Check sheet for the modelled part. Datum: model origin and axes. Units: mm. Face numbers are marked on the shaded views. A direction names the side the tool comes from. Coordinates: 2 decimals unless noted, no trailing zeros. Loops run counter-clockwise (first coordinate to the right, second up) from the corner with the lowest first, then second, coordinate; pieces in that order, holes last. Notation, with made-up numbers: M 76,-37.75 L 87,-37.75 A36 cw 87,1.25 Z; hole C 54.25,66 d4. An arc over 180 degrees is marked long. Return JSON: item names as keys, results as strings.
from build123d import *

# Parameters (mm, degrees)
SKETCH_W        = 50
SKETCH_H        = 50
SKETCH_R        = 4.56572
PAD_DEPTH       = 20
SKETCH001_W     = 35.718838
SKETCH001_H     = 17.102667
POCKET_DEPTH    = 10
POCKET001_DEPTH = 10


with BuildPart() as part:
    # Sketch → Pad (new body)
    with BuildSketch(Plane.XY):
        Rectangle(SKETCH_W, SKETCH_H)
        with Locations((-12.739399, -12.190962)):
            Circle(SKETCH_R, mode=Mode.SUBTRACT)
    extrude(amount=-PAD_DEPTH)

    # Sketch001 → Pocket (cut)
    with BuildSketch(Plane.XY):
        with Locations((-0.828983, 8.449547)):
            Rectangle(SKETCH001_W, SKETCH001_H)
    extrude(amount=-POCKET_DEPTH, mode=Mode.SUBTRACT)

    # Sketch002 → Pocket001 (cut)
    with BuildSketch(Plane.XY):
        with BuildLine():
            ThreePointArc((10.613772, -5.440841), (3.942315, -5.985276), (4.48675, -12.656733))
            Line((4.48675, -12.656733), (12.984974, -19.872584))
            ThreePointArc((12.984974, -19.872584), (19.656431, -19.328148), (19.111996, -12.656692))
            Line((10.613772, -5.440841), (19.111996, -12.656692))
        make_face()
    extrude(amount=-POCKET001_DEPTH, mode=Mode.SUBTRACT)


with BuildPart() as part_1:
    # Clone placement: moved
    add(part.part.moved(Location((25, 25, 0))))


solid = part_1.part
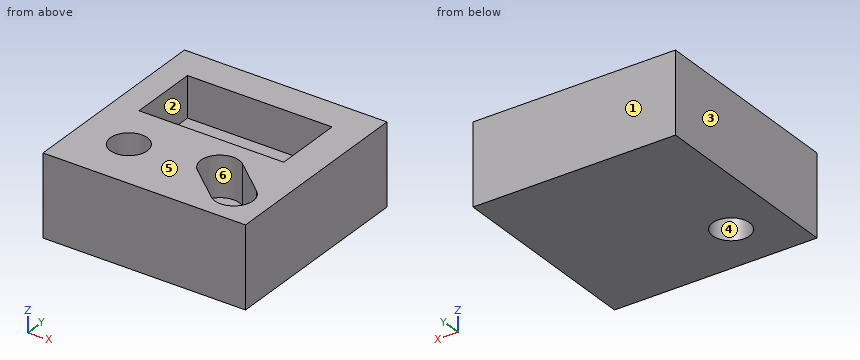
1) Section check A-A on y = 9. Record the cut outline in (x, z).
Answers:
{"outline": "M 0,-20 L 9.74,-20 L 9.74,0 L 0,0 Z; M 14.78,-20 L 50,-20 L 50,0 L 45.77,0 L 45.77,-10 L 33.42,-10 L 33.42,0 L 14.78,0 Z"}
2) Section check B-B on z = -6.75. Record the cut outline in (x, y).
Answers:
{"outline": "M 0,0 L 50,0 L 50,50 L 0,50 Z; hole M 6.31,24.9 L 42.03,24.9 L 42.03,42 L 6.31,42 Z; hole C 12.26,12.81 d9.13; hole M 29.49,12.34 L 37.98,5.13 A4.73 ccw 44.11,12.34 L 35.61,19.56 A4.73 ccw Z"}
3) Set-up check for the marked faces 5 and 6: record each of +Z, -Z, +X, -X, +Y, -Y from which the full face is reachable in a straight line by a thin tool's end or side.
Answers:
{"face 5": "+Z, +X, -X, +Y, -Y", "face 6": "+Z"}
4) Scan lines: line 1 along Y through (x, z) = (12, -9.25); line 2 along Y through (x, z) = (6.5, -3.75); line 3 along Y through (x, z) = (30.5, -9). Record each from-to range of solid material in increasing order. Write a range as [from, to].
Answers:
{"line 1": "[0, 8.25], [17.37, 24.9], [42, 50]", "line 2": "[0, 24.9], [42, 50]", "line 3": "[0, 11.48], [20.22, 24.9], [42, 50]"}
5) Go/stop test with a flat-tipped pin: pin 1 Ø5 at (x, y) = (27.5, 31) entering from +Z. Record where the tip stops, or that it passes through.
Answers:
{"pin 1": "z = -10"}
6) Draft check along Y on the marked faces 1, 2, 3 and 4. Enter one of: +Y half, -Y half, draft (parallel to the pull), parting line (faces both ways), or undercut.
Answers:
{"face 1": "+Y half", "face 2": "undercut", "face 3": "draft", "face 4": "undercut"}
7) Section check D-D on x = 19. Record the cut outline in (y, z), then the cut area to 3 significant figures.
Answers:
{"outline": "M 0,-20 L 50,-20 L 50,0 L 42,0 L 42,-10 L 24.9,-10 L 24.9,0 L 0,0 Z", "area": "829 mm²"}
8) Section check C-C on x = 10.5. Record the cut outline in (y, z), then the cut area to 3 significant figures.
Answers:
{"outline": "M 0,-20 L 8.6,-20 L 8.6,0 L 0,0 Z; M 17.02,-20 L 50,-20 L 50,0 L 42,0 L 42,-10 L 24.9,-10 L 24.9,0 L 17.02,0 Z", "area": "660 mm²"}
